Autodesk Inventor part; units mm, degrees
ref_plane "YZ Plane" through (0, 0, 0) normal (1, 0, 0) x (0, 1, 0)
ref_plane "XZ Plane" through (0, 0, 0) normal (0, 1, 0) x (-1, 0, 0)
ref_plane "XY Plane" through (0, 0, 0) normal (0, 0, 1) x (1, 0, 0)
sketch "Sketch1" plane through (0, 0, 0) normal (0, 1, 0) x (-1, 0, 0)
  line L0 (700, 350) -> (-700, 350)
  line L1 (-700, 350) -> (-700, -350)
  line L2 (-700, -350) -> (700, -350)
  line L3 (700, -350) -> (700, 350)
  line L4 (700, 350) -> (-700, -350) construction
  line L5 (-700, 350) -> (700, -350) construction
  point P0 (0, 0)
  dimension "d0" = 1400
  dimension "d1" = 700
extrude "Extrusion1" add sketch "Sketch1" along normal blind 70
sketch "Sketch2" plane through (0, 70, 0) normal (0, 1, 0) x (1, 0, 0)
  line L0 (-500, -200) -> (500, -200) construction
  line L1 (500, -200) -> (500, 200) construction
  line L2 (500, 200) -> (-500, 200) construction
  line L3 (-500, 200) -> (-500, -200) construction
  line L4 (-500, -200) -> (500, 200) construction
  line L5 (500, -200) -> (-500, 200) construction
  circle A0 centre (500, -200) radius 30
  circle A1 centre (250, -200) radius 30
  circle A2 centre (0, -200) radius 30
  circle A3 centre (-250, -200) radius 30
  circle A4 centre (-500, -200) radius 30
  circle A5 centre (500, 200) radius 30
  circle A6 centre (250, 200) radius 30
  circle A7 centre (0, 200) radius 30
  circle A8 centre (-250, 200) radius 30
  circle A9 centre (-500, 200) radius 30
  point P0 (0, 0)
  dimension "d4" = 1000
  dimension "d5" = 400
  dimension "d6" = 60
  dimension "d9" = 250
  dimension "d12" = 400
extrude "Extrusion2" cut sketch "Sketch2" against normal blind 20
sketch "Sketch3" plane through (0, 0, 0) normal (0, -1, 0) x (1, 0, 0)
  line L0 (700, 350) -> (700, -350)
  line L1 (-700, 350) -> (700, 350)
  line L2 (-700, -350) -> (-700, 350)
  line L3 (700, -350) -> (-700, -350)
  line L4 (-685, 335) -> (685, 335)
  line L5 (685, 335) -> (685, -335)
  line L6 (685, -335) -> (-685, -335)
  line L7 (-685, -335) -> (-685, 335)
  point P0 (0, 0)
  dimension "d17" = 15
extrude "Extrusion3" cut sketch "Sketch3" against normal blind 20
sketch "Sketch4" plane through (-700, 70, -350) normal (-1, 0, 0) x (0, 0, 1)
  line L0 (125, 0) -> (575, 0)
  line L1 (575, 0) -> (575, -70)
  line L2 (575, -70) -> (125, -70)
  line L3 (125, -70) -> (125, 0)
  line L4 (125, 0) -> (575, -70) construction
  line L5 (575, 0) -> (125, -70) construction
  line L6 (0, 0) -> (700, 0)
  line L7 (685, -70) -> (15, -70)
  line L8 (350, -35) -> (350, -70) construction
  dimension "d20" = 450
extrude "Extrusion4" add sketch "Sketch4" along normal blind 15 and the other way blind 15
sketch "Sketch5" plane through (0, 0, 0) normal (0, -1, 0) x (1, 0, 0)
  line L0 (-715, 225) -> (-715, -225) construction
  line L1 (-715, 0) -> (700, 0) construction
  line L2 (700, 350) -> (700, -350) construction
  line L3 (-660, 300) -> (-360, 300) construction
  line L4 (-360, 300) -> (-360, -300) construction
  line L5 (-360, -300) -> (-660, -300) construction
  line L6 (-660, -300) -> (-660, 300) construction
  line L7 (-660, 300) -> (-360, -300) construction
  line L8 (-360, 300) -> (-660, -300) construction
  line L9 (-370, 290) -> (-650, 290)
  line L10 (-650, 290) -> (-650, -290)
  line L11 (-650, -290) -> (-370, -290)
  line L12 (-370, -290) -> (-370, 290)
  line L13 (-320, 300) -> (-20, 300) construction
  line L14 (-20, 300) -> (-20, -300) construction
  line L15 (-20, -300) -> (-320, -300) construction
  line L16 (-320, -300) -> (-320, 300) construction
  line L17 (-320, 300) -> (-20, -300) construction
  line L18 (-20, 300) -> (-320, -300) construction
  line L19 (-30, 290) -> (-310, 290)
  line L20 (-310, 290) -> (-310, -290)
  line L21 (-310, -290) -> (-30, -290)
  line L22 (-30, -290) -> (-30, 290)
  line L23 (20, 300) -> (320, 300) construction
  line L24 (320, 300) -> (320, -300) construction
  line L25 (320, -300) -> (20, -300) construction
  line L26 (20, -300) -> (20, 300) construction
  line L27 (20, 300) -> (320, -300) construction
  line L28 (320, 300) -> (20, -300) construction
  line L29 (310, 290) -> (30, 290)
  line L30 (30, 290) -> (30, -290)
  line L31 (30, -290) -> (310, -290)
  line L32 (310, -290) -> (310, 290)
  line L33 (360, 300) -> (660, 300) construction
  line L34 (660, 300) -> (660, -300) construction
  line L35 (660, -300) -> (360, -300) construction
  line L36 (360, -300) -> (360, 300) construction
  line L37 (360, 300) -> (660, -300) construction
  line L38 (660, 300) -> (360, -300) construction
  line L39 (650, 290) -> (370, 290)
  line L40 (370, 290) -> (370, -290)
  line L41 (370, -290) -> (650, -290)
  line L42 (650, -290) -> (650, 290)
  line L43 (0, 0) -> (0, 331.4551) construction
  point P0 (-510, 0)
  point P1 (-170, 0)
  point P2 (170, 0)
  point P3 (510, 0)
  dimension "d25" = 300
  dimension "d26" = 600
  dimension "d27" = 10
  dimension "d30" = 340
extrude "Extrusion5" add sketch "Sketch5" along normal blind 20
sketch "Sketch6" plane through (0, -20, 0) normal (0, -1, 0) x (1, 0, 0)
  line L0 (-650, 290) -> (-650, -290) construction
  line L1 (-650, -290) -> (-370, -290) construction
  line L2 (-370, -290) -> (-370, 290) construction
  line L3 (-370, 290) -> (-650, 290) construction
  line L4 (-310, 290) -> (-310, -290) construction
  line L5 (-310, -290) -> (-30, -290) construction
  line L6 (-30, -290) -> (-30, 290) construction
  line L7 (-30, 290) -> (-310, 290) construction
  line L8 (30, 290) -> (30, -290) construction
  line L9 (30, -290) -> (310, -290) construction
  line L10 (310, -290) -> (310, 290) construction
  line L11 (310, 290) -> (30, 290) construction
  line L12 (370, 290) -> (370, -290) construction
  line L13 (370, -290) -> (650, -290) construction
  line L14 (650, -290) -> (650, 290) construction
  line L15 (650, 290) -> (370, 290) construction
  line L16 (-360, 300) -> (-360, -300)
  line L17 (-360, -300) -> (-660, -300)
  line L18 (-660, -300) -> (-660, 300)
  line L19 (-660, 300) -> (-360, 300)
  line L20 (-320, -300) -> (-320, 300)
  line L21 (-320, 300) -> (-20, 300)
  line L22 (-20, 300) -> (-20, -300)
  line L23 (-20, -300) -> (-320, -300)
  line L24 (20, -300) -> (20, 300)
  line L25 (20, 300) -> (320, 300)
  line L26 (320, 300) -> (320, -300)
  line L27 (320, -300) -> (20, -300)
  line L28 (360, -300) -> (360, 300)
  line L29 (360, 300) -> (660, 300)
  line L30 (660, 300) -> (660, -300)
  line L31 (660, -300) -> (360, -300)
  point P0 (0, 0)
  dimension "d37" = 10
  dimension "d38" = 10
  dimension "d39" = 10
  dimension "d40" = 10
extrude "Extrusion6" add sketch "Sketch6" along normal blind 10
sketch "Sketch7" plane through (-650, 0, 290) normal (0, 0, 1) x (1, 0, 0)
  line L0 (280, -20) -> (0, -20) construction
  line L1 (140, -20) -> (140, 0) construction
  line L2 (1335, 0) -> (-35, 0) construction
  circle A0 centre (140, -10) radius 5
  circle A1 centre (480, -10) radius 5
  circle A2 centre (820, -10) radius 5
  circle A3 centre (1160, -10) radius 5
  point P0 (650, 0)
  dimension "d43" = 10
  dimension "d46" = 340
extrude "Extrusion7" cut sketch "Sketch7" against normal blind 20
sketch "Sketch8" plane through (-370, 0, -290) normal (0, 0, -1) x (-1, 0, 0)
  circle A0 centre (140, -10) radius 5
  circle A1 centre (-200, -10) radius 5
  circle A2 centre (-540, -10) radius 5
  circle A3 centre (-880, -10) radius 5
  point P0 (-370, 0)
extrude "Extrusion8" cut sketch "Sketch8" against normal blind 20
sketch "Sketch9" plane through (-715, 70, -350) normal (-1, 0, 0) x (0, 0, 1)
  line L0 (700, -50) -> (0, -50)
  circle A0 centre (180.6783, -50) radius 7.5
  circle A1 centre (259.2358, -18.1737) radius 7.5
  circle A2 centre (358.3679, -32.2018) radius 7.5
  circle A3 centre (497.714, -32.2018) radius 7.5
  circle A4 centre (436.9255, -50) radius 7.5
  circle A5 centre (436.9255, -18.1737) radius 7.5
  point P0 (350, -70)
  dimension "d55" = 15
  dimension "d56" = 15
  dimension "d57" = 15
  dimension "d58" = 15
  dimension "d59" = 15
  dimension "d60" = 15
extrude "Extrusion9" add sketch "Sketch9" along normal blind 10
sketch "Sketch10" plane through (-700, 70, 350) normal (0, 0, 1) x (1, 0, 0)
  line L0 (0, -50) -> (0, 0) construction
  line L1 (0, -25) -> (1400, -25) construction
  line L2 (1400, -50) -> (1400, 0) construction
  line L3 (110, -25) -> (610, -25) construction
  line L4 (110, -35) -> (610, -35)
  line L5 (610, -15) -> (110, -15)
  arc A0 (110, -15) -> (110, -35) centre (110, -25) ccw
  arc A1 (610, -35) -> (610, -15) centre (610, -25) ccw
  line L6 (700, -70) -> (700, 0) construction
  line L7 (670, 0) -> (730, 0) construction
  line L8 (1290, -35) -> (790, -35)
  line L9 (790, -15) -> (1290, -15)
  arc A2 (1290, -35) -> (1290, -15) centre (1290, -25) ccw
  arc A3 (790, -15) -> (790, -35) centre (790, -25) ccw
  point P0 (360, -25)
  dimension "d63" = 20
  dimension "d64" = 500
  dimension "d65" = 360
extrude "Extrusion10" add sketch "Sketch10" along normal blind 10
equation "\"d9\" = 0.25 * d4"
equation "\"d12\" = d5"
properties part number "SACMI PH1500 30X60 DIE SET TOP"
The listing builds one solid part. Answer for the finished solid, in the listing's coordinates (mm). A direction names the side the tool comes from. Coordinates: 2 decimals unless noted, no trailing zeros. Write each loop counter-clockwise with the first axis right and the second up, starting at its lowest first coordinate (ties: lowest second). Pieces come first, ordered by that corner, then holes. Notation, with made-up numbers: M 86.5,-36.5 L 101.5,-36.5 A18 cw 101.5,-2.5 Z; hole C 83,55.25 d2. An arc over 180 degrees is marked long. Use a Markdown table: item, result. Add a question column.
1. Which of the six approach directions +Z, -Z, +X, -X, +Y, -Y give full straight-line access (tool end or side, diameter ignored) to faces 5 (the flat face through (508, -30, 4)), 6 (the cylindrical face through (-6.503, 60.14, -170.713))?
2. Straight lines are drawn through the part: line 1 along X through (y, z) = (-9, -48.5); line 2 along X through (y, z) = (63, 200); line 3 along X through (y, z) = (-21, 282.5). For each, find the intervals that lie inside material, in ascending order. Write a range as [from, to].
3. Given P1, Ø8, axis at x = 510, y = -10, coming from the -Z side; P2, Ø16, axis at x = 567, y = -14.5, coming from the +Z side; P3, Ø11.5, axis at x = 170, y = -10, coming from the -Z side, each flat-ended and moving along its own axis, determine where each tip first touches the part or whether it passes through.
4. For a pull along X with two mould halves and no side action, classify faces 1 (the flat face through (-512, -30, 4)), 2 (the flat face through (0, 50, -200)), 3 (the flat face through (-500, 50, -200)), 4 (the flat face through (-715, 35, -3)) as +X half, -X half, draft (parallel to the pull), parting line (faces both ways), or undercut.
5. Section A-A (x = 0) is taken. Give the vertices of the cut face in (y, z).
6. Section B-B (x = 250) is taken. Give the vertices of the cut face in (y, z), plus the area to 3 significant figures.
Data:
| question | item | result |
|---|---|---|
| 1 | face 5 | +Z, -Z, +X, -X, -Y |
| 1 | face 6 | +Y |
| 2 | line 1 | x = [-650, -370], [-310, -30], [30, 310], [370, 650] |
| 2 | line 2 | x = [-715, -530], [-470, -280], [-220, -30], [30, 220], [280, 470], [530, 700] |
| 2 | line 3 | x = [-660, -360], [-320, -20], [20, 320], [360, 660] |
| 3 | P1 | stops at z = -270 |
| 3 | P2 | stops at z = 300 |
| 3 | P3 | stops at z = -290 |
| 4 | face 1 | draft |
| 4 | face 2 | undercut |
| 4 | face 3 | undercut |
| 4 | face 4 | -X half |
| 5 | outline | M 0,-335 L 20,-335 L 20,-350 L 70,-350 L 70,-230 L 50,-230 L 50,-170 L 70,-170 L 70,170 L 50,170 L 50,230 L 70,230 L 70,350 L 20,350 L 20,335 L 0,335 Z |
| 6 | outline | M -30,-300 L -20,-300 L -20,-290 L 0,-290 L 0,-335 L 20,-335 L 20,-350 L 70,-350 L 70,-230 L 50,-230 L 50,-170 L 70,-170 L 70,170 L 50,170 L 50,230 L 70,230 L 70,350 L 55,350 L 55,360 L 35,360 L 35,350 L 20,350 L 20,335 L 0,335 L 0,290 L -20,290 L -20,300 L -30,300 Z |
| 6 | area | 63,800 mm2 |
